Source: CAD feature listing. Evaluate the final solid. Frame: model axes, mm. Face numbers are marked on the shaded views. A direction names the side the tool comes from. Round coordinates to 2 decimals unless told otherwise and drop trailing zeros. Loops run counter-clockwise (first coordinate to the right, second up) from the corner with the lowest first, then second, coordinate; pieces in that order, holes last. Notation, with made-up numbers: M 10,80.25 L 29,80.25 A18 ccw 29,87.25 Z; hole C 43.5,28.5 d10. An arc over 180 degrees is marked long. Answer as CSV lines item,"result". Start each with the question number.
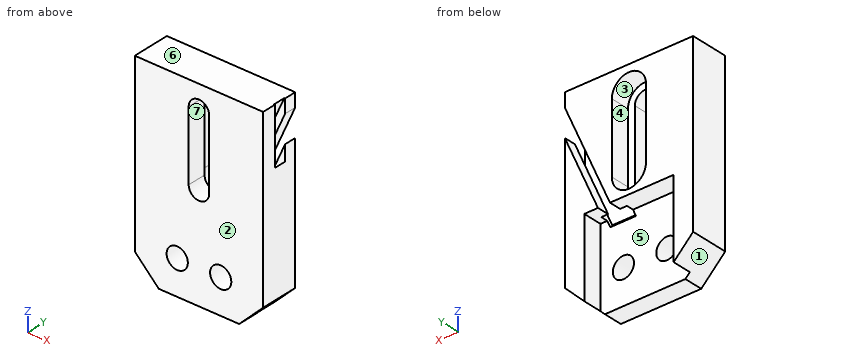
```python
from build123d import *

# Parameters (mm, degrees)
SKETCH1_W                                  = 18.75
SKETCH1_H                                  = 29.05
BOSS_EXTRUDE1_DEPTH                        = 5.55
MICROSWITCHCUTSKETCH2_W                    = 13.05
MICROSWITCHCUTSKETCH2_H                    = 12.05
MICROSWITCHCUT_EXTRUDE1_DEPTH              = 2.8
MICROSWITCHMOUNTINGHOLESSKETCH3_R          = 1.55
MICROSWITCHMOUNTINGHOLESCUT_EXTRUDE2_DEPTH = 3.1
SLIDINGMOUNTHOLECUT_EXTRUDE3_DEPTH         = 36.018102461
CHAMFER1_SIZE                              = 3.5
SLIDINGMOUNTHOLEBORECUT_EXTRUDE4_DEPTH     = 2.8
THINCABLECUT_EXTRUDE5_DEPTH                = 1.75
THICKCABLECUT_EXTRUDE6_DEPTH               = 1.75
CHAMFER2_SIZE                              = 1


with BuildPart() as part:
    # Sketch1 → Boss-Extrude1 (new body)
    with BuildSketch(Plane(origin=(0, 0, 0), x_dir=(1, 0, 0), z_dir=(0, 1, 0))):
        with Locations((9.375, 14.525)):
            Rectangle(SKETCH1_W, SKETCH1_H)
    extrude(amount=BOSS_EXTRUDE1_DEPTH)

    # MicroSwitchCutSketch2 → MicroSwitchCut-Extrude1 (cut)
    with BuildSketch(Plane(origin=(0, 5.55, 0), x_dir=(1, 0, 0), z_dir=(0, 1, 0))):
        with Locations((9.375, 23.025)):
            Rectangle(MICROSWITCHCUTSKETCH2_W, MICROSWITCHCUTSKETCH2_H)
    extrude(amount=-MICROSWITCHCUT_EXTRUDE1_DEPTH, mode=Mode.SUBTRACT)

    # MicroSwitchMountingHolesSketch3 → MicroSwitchMountingHolesCut-Extrude2 (cut)
    with BuildSketch(Plane(origin=(0, 2.75, 0), x_dir=(1, 0, 0), z_dir=(0, 1, 0))):
        with Locations(Location((6.2, 24, 0), (0, 0, 270))):
            Circle(MICROSWITCHMOUNTINGHOLESSKETCH3_R)
        with Locations(Location((12.55, 24, 0), (0, 0, 270))):
            Circle(MICROSWITCHMOUNTINGHOLESSKETCH3_R)
    extrude(amount=-MICROSWITCHMOUNTINGHOLESCUT_EXTRUDE2_DEPTH, mode=Mode.SUBTRACT)

    # GantryMountSlotSketch4 → SlidingMountHoleCut-Extrude3 (cut, through all)
    with BuildSketch(Plane(origin=(0, 5.55, 0), x_dir=(1, 0, 0), z_dir=(0, 1, 0))):
        with BuildLine():
            Line((10.875, 13.765586377), (10.875, 3.550728623))
            ThreePointArc((10.875, 3.550728623), (9.375, 2.050728623), (7.875, 3.550728623))
            Line((7.875, 3.550728623), (7.875, 13.765586377))
            ThreePointArc((7.875, 13.765586377), (9.375, 15.265586377), (10.875, 13.765586377))
        make_face()
    extrude(amount=-SLIDINGMOUNTHOLECUT_EXTRUDE3_DEPTH, mode=Mode.SUBTRACT)

    # Chamfer1
    chamfer1_edges = [part.edges().sort_by_distance(p)[0] for p in [
        (18.75, 2.775, -29.05),
        (0, 2.775, -29.05),
    ]]
    chamfer(chamfer1_edges, length=CHAMFER1_SIZE)

    # Sketch2 → SlidingMountHoleBoreCut-Extrude4 (cut)
    with BuildSketch(Plane(origin=(0, 5.55, 0), x_dir=(1, 0, 0), z_dir=(0, 1, 0))):
        with BuildLine():
            Line((6.875, 3.550728623), (6.875, 13.765586377))
            ThreePointArc((6.875, 13.765586377), (9.375, 16.265586377), (11.875, 13.765586377))
            Line((11.875, 13.765586377), (11.875, 3.550728623))
            ThreePointArc((11.875, 3.550728623), (9.375, 1.050728623), (6.875, 3.550728623))
        make_face()
    extrude(amount=-SLIDINGMOUNTHOLEBORECUT_EXTRUDE4_DEPTH, mode=Mode.SUBTRACT)

    # Sketch3 → ThinCableCut-Extrude5 (cut)
    with BuildSketch(Plane(origin=(0, 5.55, 0), x_dir=(1, 0, 0), z_dir=(0, 1, 0))):
        Polygon((12.15, 17), (18.75, 2), (18.75, 5.977272727), (13.9, 17), align=None)
    extrude(amount=-THINCABLECUT_EXTRUDE5_DEPTH, mode=Mode.SUBTRACT)

    # Sketch4 → ThickCableCut-Extrude6 (cut)
    with BuildSketch(Plane(origin=(0, 3.8, 0), x_dir=(1, 0, 0), z_dir=(0, 1, 0))):
        Polygon((11.15, 17), (18.75, -0.272727273), (18.75, 8.25), (14.9, 17), align=None)
    extrude(amount=-THICKCABLECUT_EXTRUDE6_DEPTH, mode=Mode.SUBTRACT)

    # Chamfer2
    # the kernel refuses this chamfer: 1 mm, written as the material it takes off along each edge
    with BuildSketch(Plane(origin=(17.471682988, 2.75, -17), x_dir=(0, 0.02749587661058651, -0.9996219169112968), z_dir=(-1, 0, 0))) as chamfer2_piece_1_section:
        Polygon((CHAMFER2_SIZE * 0.999621916911, CHAMFER2_SIZE * 0.0274958766106), (-CHAMFER2_SIZE * 0.0274958766106, CHAMFER2_SIZE * 0.999621916911), (0, 0), align=None)
    chamfer2_piece_1 = extrude(amount=8.893365976, mode=Mode.PRIVATE)
    chamfer2_piece_1 = split(chamfer2_piece_1, bisect_by=Plane(origin=(12.868179487, 2.05, -17.356410256), z_dir=(0, 1, 0)), keep=Keep.TOP, mode=Mode.PRIVATE)
    chamfer2_piece_1 = split(chamfer2_piece_1, bisect_by=Plane(origin=(11.297301471, 2.462820513, -16.665223929), z_dir=(0.9153150324227658, 0, -0.40273861426601665)), keep=Keep.TOP, mode=Mode.PRIVATE)
    chamfer2_piece_1 = split(chamfer2_piece_1, bisect_by=Plane(origin=(14.439057503, 2.462820513, -18.047596583), z_dir=(-0.9153150324227658, 0, 0.40273861426601687)), keep=Keep.TOP, mode=Mode.PRIVATE)
    add(chamfer2_piece_1, mode=Mode.SUBTRACT)


solid = part.part
```
1) Section B-B, the plane y = 4.7. Return loops of the section in (x, z) (3 decimals).
2) Access query for the marked faces 4, 5, 6 and 7. Directions: +Z, -Z, +X, -X, +Y, -Y. A direction counts if a zero-diameter tool reaches every point of the face in a straight line with its end or side. Return the directions, or none.
3) Contact query for flat-ended pins moving along their axis: pin 1 Ø3 at (x, z) = (6.2, -24) entering from -Y; pin 2 Ø6 at (x, z) = (10.5, -23) entering from +Y; pin 3 Ø1 at (x, y) = (15, 4) entering from -Z. Output: stop coordinate, or through.
4) Ray query, line 1 along X through (y, z) = (1.45, -24); line 2 along X through (y, z) = (4.2, -24); line 3 along Y through (x, z) = (5.5, -21.75). Return the intervals inside material, ascending.
5) Section D-D, the plane x = 9.75. Return loops of the section in (y, z).
6) Section C-C, the plane z = -12.75. Return loops of the section in (x, y) (3 decimals), and give its area (3 significant figures).
7) Section A-A, the plane z = -7.75. Return loops of the section in (x, y) (3 decimals), and give its area (3 significant figures).
8) Mould query, pull axis X, two halves, no side actions, for the marked faces 1, 2 and 3. Classes: pulls with the +X half, pulls with the -X half, needs draft (parallel to the pull), parting line crosses it, or undercut.
Findings below:
1,outline,"M 0,-25.55 L 2.85,-28.4 L 2.85,-17 L 12.15,-17 L 18.75,-2 L 18.75,0 L 0,0 Z; M 13.9,-17 L 15.9,-17 L 15.9,-28.4 L 18.75,-25.55 L 18.75,-5.977 Z; hole M 6.875,-13.766 A2.5 ccw 11.875,-13.766 L 11.875,-3.551 A2.5 ccw 6.875,-3.551 Z"
2,face 4,"+Y"
2,face 5,"-Z, +Y"
2,face 6,"+Z, +X, -X, +Y, -Y"
2,face 7,"+Y, -Y"
3,pin 1,"through"
3,pin 2,"y = 2.75"
3,pin 3,"z = -17"
4,line 1,"0 to 4.65, 7.75 to 11, 14.1 to 18.75"
4,line 2,"0 to 2.85, 15.9 to 18.75"
4,line 3,"0 to 2.75"
5,outline,"M 0,-29.05 L 2.75,-29.05 L 2.75,-17 L 5.55,-17 L 5.55,-16.24 L 2.75,-16.24 L 2.75,-15.22 L 0,-15.22 Z; M 0,-2.1 L 2.75,-2.1 L 2.75,-1.08 L 5.55,-1.08 L 5.55,0 L 0,0 Z"
6,outline,"M 0,0 L 7.875,0 L 7.875,2.75 L 6.875,2.75 L 6.875,5.55 L 0,5.55 Z; M 10.875,0 L 18.75,0 L 18.75,5.55 L 15.77,5.55 L 15.77,3.8 L 16.77,3.8 L 16.77,2.05 L 13.02,2.05 L 13.02,3.8 L 14.02,3.8 L 14.02,5.55 L 11.875,5.55 L 11.875,2.75 L 10.875,2.75 Z"
6,area,"72.2 mm²"
7,outline,"M 0,0 L 7.875,0 L 7.875,2.75 L 6.875,2.75 L 6.875,5.55 L 0,5.55 Z; M 10.875,0 L 18.75,0 L 18.75,2.05 L 15.22,2.05 L 15.22,3.8 L 16.22,3.8 L 16.22,5.55 L 11.875,5.55 L 11.875,2.75 L 10.875,2.75 Z; M 17.97,3.8 L 18.75,3.8 L 18.75,5.55 L 17.97,5.55 Z"
7,area,"72.6 mm²"
8,face 1,"pulls with the -X half"
8,face 2,"needs draft"
8,face 3,"undercut"
